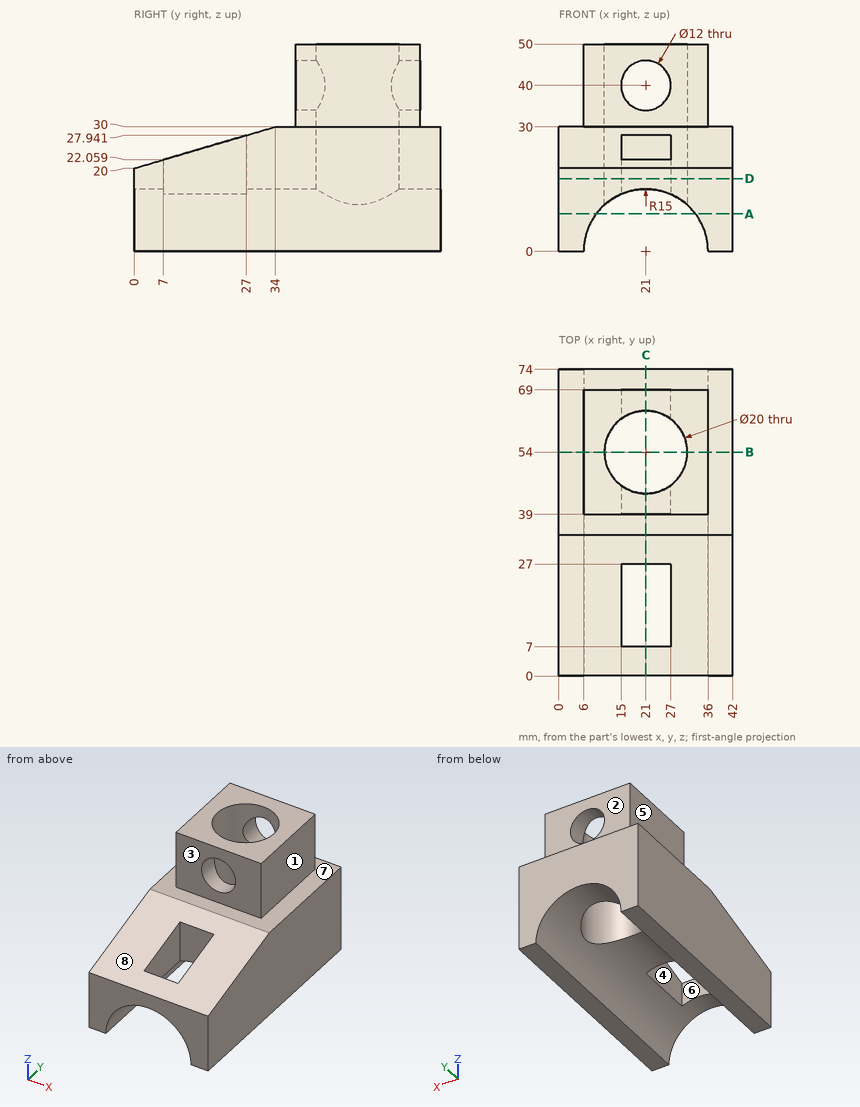
Can you work these out from the drawing? Everything is in mm from the part's minimum corner. A direction names the side the tool comes from. Round coordinates to 2 decimals unless told otherwise and drop trailing zeros. Loops run counter-clockwise (first coordinate to the right, second up) from the corner with the lowest first, then second, coordinate; pieces in that order, holes last. Notation, with made-up numbers: (-27.75, -36) - (26.25, -36) arc R17 cw to (26.25, -20) - close; hole circle Ø6 at (78.25, -27.5). An arc over 180 degrees is marked (long way). Write item = value, one per line. Start each with the question number.
(1) For the marked faces 1, 2, 3, 4 and 5, which set-ups out of +Z, -Z, +X, -X, +Y, -Y let a thin tool reach every point of the face, with its end or its side?
(2) For P1, Ø3, axis at x = 9, z = 39, coming from the +Y side; P2, Ø22, axis at x = 28, z = 42.5, coming from the -Y side; P3, Ø2, axis at y = 44, z = 43, coming from the +X side, each with a flat end and sliding along its axis, tell me the tip position at first contact or that it passes through.
(3) If we section it at D-D (z = 17.5): Please give me the cut outline in (x, y), and give its area (3 significant figures).
(4) If we section it at A-A (z = 9): Please give me the cut outline in (x, y).
(5) If we section it at C-C (x = 21): Please give me the cut outline in (y, z).
(6) If we section it at B-B (y = 54): Please give me the cut outline in (x, z).
(7) If we mould it in two halves opening along Y, with no side actions, what happens to the marked faces 6, 7 and 8? For each: released by +Y, released by -Y, zero draft, split by the parting line, or undercut.
(8) If I drill on probe 1 along X at (y, z) = (8.5, 19); probe 2 along Y at (x, z) = (21, 27); probe 3 along Y at (x, z) = (29, 32.5), over which ranges is the centre line in solid material (lowest first)? Write a range as [from, to].
Ans:
q1.face_1 = +Z, +X, +Y, -Y
q1.face_2 = +Z, +X, -X, +Y
q1.face_3 = +Z, +X, -X, -Y
q1.face_4 = +Z, -Z
q1.face_5 = +Z, -X, +Y, -Y
q2.P1 = 69
q2.P2 = 39
q2.P3 = 36
q3.outline = (0, 0) - (42, 0) - (42, 74) - (0, 74) - close; hole circle Ø20 at (21, 54); hole (15, 7) - (27, 7) - (27, 27) - (15, 27) - close
q3.area = 2,550 mm²
q4.outline = (0, 0) - (9, 0) - (9, 74) - (0, 74) - close; (33, 0) - (42, 0) - (42, 74) - (33, 74) - close
q5.outline = (0, 15) - (7, 15) - (7, 22.06) - (0, 20) - close; (27, 15) - (44, 15) - (44, 34) - (39, 34) - (39, 30) - (34, 30) - (27, 27.94) - close; (39, 46) - (44, 46) - (44, 50) - (39, 50) - close; (64, 15) - (74, 15) - (74, 30) - (69, 30) - (69, 34) - (64, 34) - close; (64, 46) - (69, 46) - (69, 50) - (64, 50) - close
q6.outline = (0, 0) - (6, 0) arc R15 cw to (11, 11.18) - (11, 50) - (6, 50) - (6, 30) - (0, 30) - close; (31, 11.18) arc R15 cw to (36, 0) - (42, 0) - (42, 30) - (36, 30) - (36, 50) - (31, 50) - close
q7.face_6 = undercut
q7.face_7 = zero draft
q7.face_8 = released by -Y
q8.probe_1 = [0, 15], [27, 42]
q8.probe_2 = [27, 44], [64, 74]
q8.probe_3 = [39, 48], [60, 69]
